The model under review builds one solid part; all positions refer to its coordinate system, in mm. Round coordinates to 2 decimals unless told otherwise and drop trailing zeros. Loops run counter-clockwise (first coordinate to the right, second up) from the corner with the lowest first, then second, coordinate; pieces in that order, holes last. Notation, with made-up numbers: (36, 27) -> (63, 27) arc R18 cw to (63, 57) -> close; hole circle Ø10 at (-22, -27.5). An arc over 180 degrees is marked (long way). Use a Markdown table: item, result. Add a question column.
1) Consider section C-C on x = -41.5. Give the boundary of the cut face in (y, z).
2) Consider section A-A on y = 3. Give the boundary of the cut face in (x, z), plus the area to 4 significant figures.
3) Consider section B-B on x = 37.33. Give the boundary of the cut face in (y, z), plus the area to 3 significant figures.
4) Wall thickness on probe 1 along Y at (x, z) = (-5, 1.3); probe 2 along Y at (x, z) = (-41.5, 1.2); probe 3 along Y at (x, z) = (37.33, 0.45): over which ranges is each line inside the solid? List them lowest first.
from build123d import *

# Parameters (mm, degrees)
SKETCH1_W                  = 92.5
SKETCH1_H                  = 92.5
BOSS_EXTRUDE1_DEPTH        = 1.5
F_3_1_3_1_DIAMETER_HOLE1_D = 3.1
F_2_5_2_5_DIAMETER_HOLE1_D = 2.5


with BuildPart() as part:
    # Sketch1 → Boss-Extrude1 (new body)
    with BuildSketch(Plane.XY):
        Rectangle(SKETCH1_W, SKETCH1_H)
    extrude(amount=BOSS_EXTRUDE1_DEPTH)

    # Ø3.1 (3.1) Diameter Hole1 (through all)
    with Locations(Plane.XY.offset(1.5)):
        with Locations((-41.5, 41.5), (41.5, 41.5), (37.33, -44.05), (-41.5, -41.5)):
            Hole(F_3_1_3_1_DIAMETER_HOLE1_D / 2)

    # Ø2.5 (2.5) Diameter Hole1 (through all)
    with Locations(Plane(origin=(0, 0, 0), x_dir=(-1, 0, 0), z_dir=(0, 0, -1))):
        with Locations((19.704975955, 3), (19.704975955, -3), (12.454975955, -3), (12.454975955, 3), (5.204975955, 3), (5.204975955, -3), (-29.795024045, 12.502014748), (-29.795024045, -12.501777911)):
            Hole(F_2_5_2_5_DIAMETER_HOLE1_D / 2)


solid = part.part
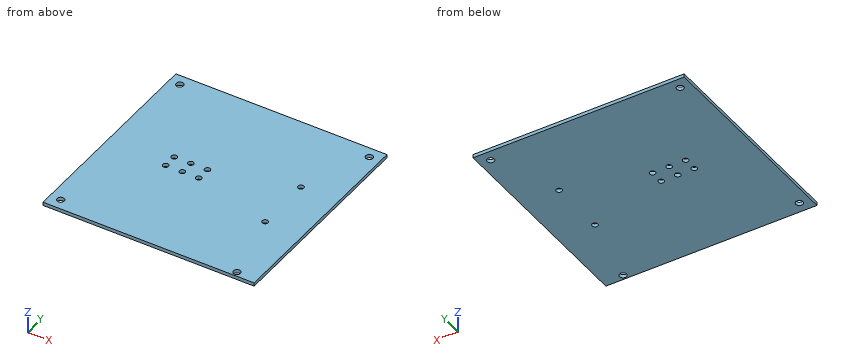
Result set:
| question | item | result |
|---|---|---|
| 1 | outline | (-46.25, 0) -> (-43.05, 0) -> (-43.05, 1.5) -> (-46.25, 1.5) -> close; (-39.95, 0) -> (39.95, 0) -> (39.95, 1.5) -> (-39.95, 1.5) -> close; (43.05, 0) -> (46.25, 0) -> (46.25, 1.5) -> (43.05, 1.5) -> close |
| 2 | outline | (-46.25, 0) -> (-20.95, 0) -> (-20.95, 1.5) -> (-46.25, 1.5) -> close; (-18.45, 0) -> (-13.7, 0) -> (-13.7, 1.5) -> (-18.45, 1.5) -> close; (-11.2, 0) -> (-6.45, 0) -> (-6.45, 1.5) -> (-11.2, 1.5) -> close; (-3.95, 0) -> (46.25, 0) -> (46.25, 1.5) -> (-3.95, 1.5) -> close |
| 2 | area | 127.5 mm2 |
| 3 | outline | (-46.25, 0) -> (-45.6, 0) -> (-45.6, 1.5) -> (-46.25, 1.5) -> close; (-42.5, 0) -> (46.25, 0) -> (46.25, 1.5) -> (-42.5, 1.5) -> close |
| 3 | area | 134 mm2 |
| 4 | probe 1 | -46.25 to -4.23, -1.77 to 1.77, 4.23 to 46.25 |
| 4 | probe 2 | -46.25 to -43.05, -39.95 to 39.95, 43.05 to 46.25 |
| 4 | probe 3 | -46.25 to -45.6, -42.5 to 46.25 |
